Read the model definition and answer for the solid it produces. Units are mm, in the model's axes. A direction names the side the tool comes from. Coordinates: 2 decimals unless noted, no trailing zeros. Write each loop counter-clockwise with the first axis right and the second up, starting at its lowest first coordinate (ties: lowest second). Pieces come first, ordered by that corner, then holes.
(1) The part is cut by section A-A, the plane x = 0. Determine the outline of the cut face in (y, z), and give its area (3 significant figures).
(2) The part is cut by section C-C, the plane z = 0. Determine the outline of the cut face in (x, y).
(3) Given pin 1 (4 mm diameter, centred on y = 3.5, z = -3.5, fed in from -X); pin 2 (8 mm diameter, centred on x = -10, y = 7, fed in from +Z); pin 3 (1.1 mm diameter, centred on x = -10, y = 5, fed in from -Z); pin 4 (6.5 mm diameter, centred on x = 0, z = 0, fed in from -Y), each flat-ended and moving along its own axis, determine where each tip first touches the part or whether it passes through.
(4) The part is cut by section B-B, the plane y = 2. Determine the outline of the cut face in (x, z), and give its area (3 significant figures).
(5) Which of the six approach directions +Z, -Z, +X, -X, +Y, -Y give full straight-line access (tool end or side, diameter ignored) to faces 1 (the conical face through (12.38, 6.87, -0.04)), 2 (the flat face through (-7.5, 3, 5)), 3 (the flat face through (-7.2, 7, 0))?
(6) Straight lines are drawn through the part: line 1 along Z through (x, y) = (0, 10.25); line 2 along Z through (x, y) = (-10.5, 2); line 3 along Y through (x, z) = (-4.5, 5.5). For each, find the intervals that lie inside material, in ascending order.
(7) Determine the mould class of faces 4 (the flat face through (7.5, 3, -5)), 5 (the cylindrical face through (6.466, 11.314, 2.681)), 6 (the cylindrical face through (11.09, 3.45, -0.54)) for opening direction X: pulls with the +X half, pulls with the -X half, needs draft (parallel to the pull), parting line crosses it, or undercut.
(8) The part is cut by section D-D, the plane y = 9.75. Determine the outline of the cut face in (x, z).
```python
from build123d import *

# Parameters (mm, degrees)
BOSS_EXTRUDE1_DEPTH     = 7
FILLET1_R               = 2
M2X0_4_TAPPED_HOLE1_D   = 1.6
CHAMFER1_SIZE           = 0.25
SKETCH4_R               = 7
BOSS_EXTRUDE2_DEPTH     = 9
CHAMFER2_SIZE           = 0.25
M12X1_25_TAPPED_HOLE1_D = 10.8


with BuildPart() as part:
    # Sketch1 → Boss-Extrude1 (new body)
    with BuildSketch(Plane(origin=(0, 0, 0), x_dir=(1, 0, 0), z_dir=(0, 1, 0))):
        with BuildLine():
            Line((-7.5, 8), (7.5, 8))
            Line((7.5, 8), (7.5, 2))
            Line((7.5, 2), (10.5, 2))
            ThreePointArc((10.5, 2), (12.5, 0), (10.5, -2))
            Line((10.5, -2), (7.5, -2))
            Line((7.5, -2), (7.5, -8))
            Line((7.5, -8), (-7.5, -8))
            Line((-7.5, -8), (-7.5, -2))
            Line((-7.5, -2), (-10.5, -2))
            ThreePointArc((-10.5, -2), (-12.5, 0), (-10.5, 2))
            Line((-10.5, 2), (-7.5, 2))
            Line((-7.5, 2), (-7.5, 8))
        make_face()
    extrude(amount=BOSS_EXTRUDE1_DEPTH)

    # Fillet1
    fillet1_edges = [part.edges().sort_by_distance(p)[0] for p in [
        (7.5, 3.5, 8),
        (-7.5, 3.5, 8),
        (-7.5, 3.5, 2),
        (-7.5, 3.5, -2),
        (-7.5, 3.5, -8),
        (7.5, 3.5, -8),
        (7.5, 3.5, -2),
        (7.5, 3.5, 2),
    ]]
    fillet(fillet1_edges, radius=FILLET1_R)

    # M2x0.4 Tapped Hole1 (through all)
    with Locations(Plane(origin=(0, 7, 0), x_dir=(1, 0, 0), z_dir=(0, 1, 0))):
        with Locations((10.5, 0), (-10.5, 0)):
            Hole(M2X0_4_TAPPED_HOLE1_D / 2)

    # Chamfer1
    chamfer1_edges = [part.edges().sort_by_distance(p)[0] for p in [
        (12.5, 7, 0),
        (10, 7, -2),
        (-12.5, 7, 0),
        (-10, 7, 2),
        (7.5, 7, -5),
        (0, 7, -8),
        (7.5, 7, 5),
        (10, 7, 2),
        (-7.5, 7, -5),
        (-10, 7, -2),
        (-7.5, 7, 5),
        (0, 7, 8),
        (6.914213562, 7, 7.414213562),
        (-6.914213562, 7, 7.414213562),
        (-6.914213562, 7, -7.414213562),
        (6.914213562, 7, -7.414213562),
        (8.085786438, 7, -2.585786438),
        (-8.085786438, 7, -2.585786438),
        (-8.085786438, 7, 2.585786438),
        (8.085786438, 7, 2.585786438),
    ]]
    chamfer(chamfer1_edges, length=CHAMFER1_SIZE)

    # Sketch4 → Boss-Extrude2 (add)
    with BuildSketch(Plane(origin=(0, 7, 0), x_dir=(1, 0, 0), z_dir=(0, 1, 0))):
        Circle(SKETCH4_R)
    extrude(amount=BOSS_EXTRUDE2_DEPTH)

    # Chamfer2
    chamfer2_edges = [part.edges().sort_by_distance(p)[0] for p in [
        (-7, 16, 0),
    ]]
    chamfer(chamfer2_edges, length=CHAMFER2_SIZE)

    # M12x1.25 Tapped Hole1 (through all)
    with Locations(Plane(origin=(0, 16, 0), x_dir=(1, 0, 0), z_dir=(0, 1, 0))):
        with Locations((0, 0)):
            Hole(M12X1_25_TAPPED_HOLE1_D / 2)


solid = part.part
```
Computed:
1. outline: (0, -8) - (6.75, -8) - (7, -7.75) - (7, -7) - (15.75, -7) - (16, -6.75) - (16, -5.4) - (0, -5.4) - close; (0, 5.4) - (16, 5.4) - (16, 6.75) - (15.75, 7) - (7, 7) - (7, 7.75) - (6.75, 8) - (0, 8) - close
1. area: 65.1 mm2
2. outline: (-12.5, 0) - (-11.3, 0) - (-11.3, 7) - (-12.25, 7) - (-12.5, 6.75) - close; (-9.7, 0) - (-5.4, 0) - (-5.4, 16) - (-6.75, 16) - (-7, 15.75) - (-7, 7) - (-9.7, 7) - close; (5.4, 0) - (9.7, 0) - (9.7, 7) - (7, 7) - (7, 15.75) - (6.75, 16) - (5.4, 16) - close; (11.3, 0) - (12.5, 0) - (12.5, 6.75) - (12.25, 7) - (11.3, 7) - close
3. pin 1: stops at x = -11.82
3. pin 2: stops at z = 7.93
3. pin 3: stops at z = -2
3. pin 4: passes through
4. outline: (-10.5, -2) - (-9.5, -2) arc R2 cw to (-7.5, -4) - (-7.5, -6) arc R2 ccw to (-5.5, -8) - (5.5, -8) arc R2 ccw to (7.5, -6) - (7.5, -4) arc R2 cw to (9.5, -2) - (10.5, -2) arc R2 ccw to (10.5, 2) - (9.5, 2) arc R2 cw to (7.5, 4) - (7.5, 6) arc R2 ccw to (5.5, 8) - (-5.5, 8) arc R2 ccw to (-7.5, 6) - (-7.5, 4) arc R2 cw to (-9.5, 2) - (-10.5, 2) arc R2 ccw to start; hole circle Ø1.6 at (-10.5, 0); hole circle Ø10.8 at (0, 0); hole circle Ø1.6 at (10.5, 0)
4. area: 181 mm2
5. face 1: +X, +Y
5. face 2: +Z, -X, +Y, -Y
5. face 3: +Y
6. line 1: z = -7 to -5.4, 5.4 to 7
6. line 2: z = -2 to -0.8, 0.8 to 2
6. line 3: y = 0 to 7
7. face 4: pulls with the +X half
7. face 5: parting line crosses it
7. face 6: undercut
8. outline: circle Ø14 at (0, 0); hole circle Ø10.8 at (0, 0)
